Work out the finished part from the listing and answer in its coordinate system (mm). Coordinates: 2 decimals unless noted, no trailing zeros. Write each loop counter-clockwise with the first axis right and the second up, starting at its lowest first coordinate (ties: lowest second). Pieces come first, ordered by that corner, then holes. Notation, with made-up numbers: (-5.5, 47.5) - (25.5, 47.5) arc R24 ccw to (25.5, 66.5) - close; hole circle Ø5 at (-35, 75.25). An arc over 180 degrees is marked (long way). One line per item, written item: value.
```python
from build123d import *

# Parameters (mm, degrees)
F0_R      = 95
F1_DEPTH  = 30
F2_W      = 95
F2_H      = 95
F3_DEPTH  = 40
F4_R      = 9
F5_DEPTH  = 30
F6_R      = 5.25
F7_DEPTH  = 40
F9_DEPTH  = 24
F10_W     = 56
F10_H     = 56
F10_W_2   = 57
F10_H_2   = 5
F10_W_3   = 5
F10_H_3   = 57
F11_DEPTH = 24
F13_DEPTH = 1.2
F15_DEPTH = 8
F16_R     = 6
F17_W     = 28
F17_H     = 15
F18_DEPTH = 6
F19_R     = 11


with BuildPart() as f1:
    # F0 (on Front) → F1 (new body)
    with BuildSketch(Plane.XZ):
        Circle(F0_R)
    extrude(amount=F1_DEPTH)

    # F2 (on face) → F3 (cut)
    with BuildSketch(Plane.XZ.offset(30)):
        with Locations((-47.5, -47.5)):
            Rectangle(F2_W, F2_H)
    extrude(amount=-F3_DEPTH, mode=Mode.SUBTRACT)

    # F4 (on face) → F5 (join)
    with BuildSketch(Plane.XZ.offset(30)):
        Circle(F4_R)
    extrude(amount=-F5_DEPTH)

    # F6 (on face) → F7 (cut)
    with BuildSketch(Plane.XZ.offset(30)):
        Circle(F6_R)
    extrude(amount=-F7_DEPTH, mode=Mode.SUBTRACT)

    # F8 (on face) → F9 (cut)
    with BuildSketch(Plane(origin=(0, 0, 0), x_dir=(-1, 0, 0), z_dir=(0, 1, 0))):
        with BuildLine():
            ThreePointArc((0, -9), (6.3639610307, -6.3639610307), (9, 0))
            Line((9, 0), (5.25, 0))
            ThreePointArc((5.25, 0), (3.7123106012, -3.7123106012), (0, -5.25))
            Line((0, -5.25), (0, -9))
        make_face()
        with BuildLine():
            ThreePointArc((0, -5.25), (3.7123106012, -3.7123106012), (5.25, 0))
            Line((5.25, 0), (0, 0))
            Line((0, 0), (0, -5.25))
        make_face()
        with BuildLine():
            ThreePointArc((-5, 1.6007810594), (-3.7123106012, 3.7123106012), (-1.6007810594, 5))
            Line((-1.6007810594, 5), (-5, 5))
            Line((-5, 5), (-5, 1.6007810594))
        make_face()
        with BuildLine():
            Line((-1.6007810594, 5), (1.6007810594, 5))
            ThreePointArc((1.6007810594, 5), (0, 5.25), (-1.6007810594, 5))
        make_face()
        with BuildLine():
            Line((1.6007810594, 5), (89.8610037781, 5))
            ThreePointArc((89.8610037781, 5), (-63.6396103068, 63.6396103068), (-5, -89.8610037781))
            Line((-5, -89.8610037781), (-5, -1.6007810594))
            ThreePointArc((-5, -1.6007810594), (-5.25, 0), (-5, 1.6007810594))
            Line((-5, 1.6007810594), (-5, 5))
            Line((-5, 5), (-1.6007810594, 5))
            ThreePointArc((-1.6007810594, 5), (0, 5.25), (1.6007810594, 5))
        make_face()
        with BuildLine():
            ThreePointArc((0, -90), (63.6396103068, -63.6396103068), (90, 0))
            Line((90, 0), (9, 0))
            ThreePointArc((9, 0), (6.3639610307, -6.3639610307), (0, -9))
            Line((0, -9), (0, -90))
        make_face()
        with BuildLine():
            Line((9, 0), (90, 0))
            ThreePointArc((90, 0), (89.9652442336, 2.5009658109), (89.8610037781, 5))
            Line((89.8610037781, 5), (1.6007810594, 5))
            ThreePointArc((1.6007810594, 5), (4.2406721496, 3.0950282259), (5.25, 0))
            Line((5.25, 0), (9, 0))
        make_face()
        with BuildLine():
            ThreePointArc((-5, -89.8610037781), (-2.5009658109, -89.9652442336), (0, -90))
            Line((0, -90), (0, -9))
            Line((0, -9), (0, -5.25))
            ThreePointArc((0, -5.25), (-3.0950282259, -4.2406721496), (-5, -1.6007810594))
            Line((-5, -1.6007810594), (-5, -89.8610037781))
        make_face()
        with BuildLine():
            ThreePointArc((5.25, 0), (4.2406721496, 3.0950282259), (1.6007810594, 5))
            Line((1.6007810594, 5), (-1.6007810594, 5))
            ThreePointArc((-1.6007810594, 5), (-3.7123106012, 3.7123106012), (-5, 1.6007810594))
            Line((-5, 1.6007810594), (-5, -1.6007810594))
            ThreePointArc((-5, -1.6007810594), (-3.0950282259, -4.2406721496), (0, -5.25))
            Line((0, -5.25), (0, 0))
            Line((0, 0), (5.25, 0))
        make_face()
    extrude(amount=-F9_DEPTH, mode=Mode.SUBTRACT)

    # F10 (on face) → F11 (join)
    with BuildSketch(Plane(origin=(0, -24, 0), x_dir=(-1, 0, 0), z_dir=(0, 1, 0))):
        Polygon((33, 5), (33, 33), (-33, 33), (-33, -33), (-5, -33), (0, -33), (33, -33), (33, 0), align=None)
        Rectangle(F10_W, F10_H, mode=Mode.SUBTRACT)
        with Locations((61.5, 2.5)):
            Rectangle(F10_W_2, F10_H_2)
        with Locations((-2.5, -61.5)):
            Rectangle(F10_W_3, F10_H_3)
    extrude(amount=F11_DEPTH)

    # F12 (on face) → F13 (join)
    with BuildSketch(Plane.XZ.offset(24)):
        with BuildLine():
            Line((-28, 0), (-28, -28))
            Line((-28, -28), (0, -28))
            Line((0, -28), (0, -9))
            ThreePointArc((0, -9), (-6.3639610307, -6.3639610307), (-9, 0))
            Line((-9, 0), (-28, 0))
        make_face()
        Polygon((0, -28), (-28, -28), (-28, 0), (-33, 0), (-33, -33), (0, -33), align=None)
    extrude(amount=F13_DEPTH)

    # F14 (on face) → F15 (cut)
    with BuildSketch(Plane(origin=(0, 0, 0), x_dir=(-1, 0, 0), z_dir=(0, 1, 0))):
        Polygon((33, 33), (-33, 33), (-33, -33), (-5, -33), (-5, -28), (-28, -28), (-28, 28), (28, 28), (28, 5), (33, 5), align=None)
    extrude(amount=-F15_DEPTH, mode=Mode.SUBTRACT)

    # F16
    f16_edges = [f1.edges().sort_by_distance(p)[0] for p in [
        (-28, -12, -28),
        (28, -16, -28),
        (28, -16, 28),
        (-28, -16, 28),
    ]]
    fillet(f16_edges, radius=F16_R)

    # F17 (on face) → F18 (cut)
    with BuildSketch(Plane(origin=(0, -8, 0), x_dir=(-1, 0, 0), z_dir=(0, 1, 0))):
        with Locations((-19, -25.5)):
            Rectangle(F17_W, F17_H)
    extrude(amount=-F18_DEPTH, mode=Mode.SUBTRACT)

    # F19
    f19_edges = [f1.edges().sort_by_distance(p)[0] for p in [
        (33, -19, -33),
        (-33, -12.6, -33),
        (33, -16, 33),
        (-33, -16, 33),
    ]]
    fillet(f19_edges, radius=F19_R)


solid = f1.part
```
Item 1: Determine the mould class of faces 1 (the face through (-29.863, -12.776, -29.692)), 2 (the face through (0.4, 0, -34.7)), 3 (the face through (5, -27, 1.6)), 4 (the face through (28, -16, 0)) for opening direction Z: +Z half, -Z half, draft (parallel to the pull), parting line (faces both ways), or undercut.
Evaluation:
face 1: -Z half
face 2: draft
face 3: undercut
face 4: undercut
Item 2: Section D-D, the plane x = -18.5 is taken. Determine the outline of the cut face in (y, z), then the cut area to 3 significant figures.
Evaluation:
outline: (-30, 0) - (-25.2, 0) - (-25.2, -33) - (0, -33) - (0, -28) - (-24, -28) - (-24, 28) - (-8, 28) - (-8, 33) - (-24, 33) - (-24, 88.08) - (0, 88.08) - (0, 93.18) - (-30, 93.18) - close
area: 921 mm2
Item 3: Given pin 1 (10 mm diameter, centred on x = 13, y = -10, fed in from -Z); pin 2 (10 mm diameter, centred on y = -21.5, z = 43.5, fed in from -X); pin 3 (15 mm diameter, centred on x = -54, y = -18, fed in from -Z), each flat-ended and moving along its own axis, determine where each tip first touches the part or whether it passes through.
Evaluation:
pin 1: stops at z = -94.66
pin 2: stops at x = -86.85
pin 3: stops at z = 0
Item 4: Section C-C, the plane x = 75 is taken. Determine the outline of the cut face in (y, z).
Evaluation:
outline: (-30, -58.31) - (0, -58.31) - (0, -49.75) - (-24, -49.75) - (-24, 49.75) - (0, 49.75) - (0, 58.31) - (-30, 58.31) - close
Item 5: Section A-A, the plane y = -19 is taken. Determine the outline of the cut face in (x, z).
Evaluation:
outline: (-95, 0) - (-33, 0) - (-33, -22) arc R11 ccw to (-22, -33) - (0, -33) - (0, -95) arc R95 ccw (long way) to start; hole (-89.86, 5) - (-33, 5) - (-33, 22) arc R11 cw to (-22, 33) - (22, 33) arc R11 cw to (33, 22) - (33, -22) arc R11 cw to (22, -33) - (5, -33) - (5, -89.86) arc R90 ccw (long way) to start; hole (-28, -22) arc R6 ccw to (-22, -28) - (22, -28) arc R6 ccw to (28, -22) - (28, 22) arc R6 ccw to (22, 28) - (-22, 28) arc R6 ccw to (-28, 22) - close
Item 6: Section B-B, the plane z = -51 is taken. Determine the outline of the cut face in (x, y), then the cut area to 3 significant figures.
Evaluation:
outline: (0, -30) - (80.15, -30) - (80.15, 0) - (74.16, 0) - (74.16, -24) - (5, -24) - (5, 0) - (0, 0) - close
area: 745 mm2
Item 7: Consider probe 1 along Z at (x, y) = (-2, -14); probe 2 along Z at (x, y) = (1.5, -19.5); probe 3 along Y at (x, z) = (44, 29.5). Determine where each line is inside the solid, lowest interval first.
Evaluation:
probe 1: z = -33 to -28, 28 to 33, 89.98 to 94.98
probe 2: z = -94.99 to -28, 28 to 33, 89.99 to 94.99
probe 3: y = -30 to -24
